Design review of the part shown in the three views and the two pictorial views. Dimensions are in mm from the part's minimum x, y and z. A direction names the side the tool comes from. Give positions to 0.01 mm unless a question says otherwise; leave off trailing zeros. Loops run counter-clockwise (first coordinate to the right, second up) from the corner with the lowest first, then second, coordinate; pieces in that order, holes last. Notation, with made-up numbers: (65, 56) -> (113, 56) arc R13 cw to (113, 70) -> close; hole circle Ø6 at (74.5, -13). An arc over 180 degrees is marked (long way). One line per question, with ' | ' between items. Start each with the question number.
(1) Wall thickness on probe 1 along Y at (x, z) = (20, 3.75); probe 2 along Y at (x, z) = (19, 2.5); probe 3 along X at (y, z) = (3.5, 1.5): over which ranges is each line inside the solid? List them lowest first.
(2) Consider section D-D (z = 8.75). Write out the cut boundary in (x, y), and give its area (3 significant figures).
(3) Draft analysis for pull direction Y (two halves, no side actions). For the marked faces 3, 4, 5 and 6, state which applies: +Y half, -Y half, draft (parallel to the pull), parting line (faces both ways), or undercut.
(4) Consider section A-A (z = 1.25). Write out the cut boundary in (x, y), and give its area (3 significant figures).
(5) Consider section C-C (y = 4). Write out the cut boundary in (x, z), and give its area (3 significant figures).
(6) Tool access review of the marked faces 1 and 2: name each direction out of +Z, -Z, +X, -X, +Y, -Y from which nothing blocks a thin tool from reaching the whole face with its end or side.
(7) Consider section B-B (x = 4). Write out the cut boundary in (y, z).
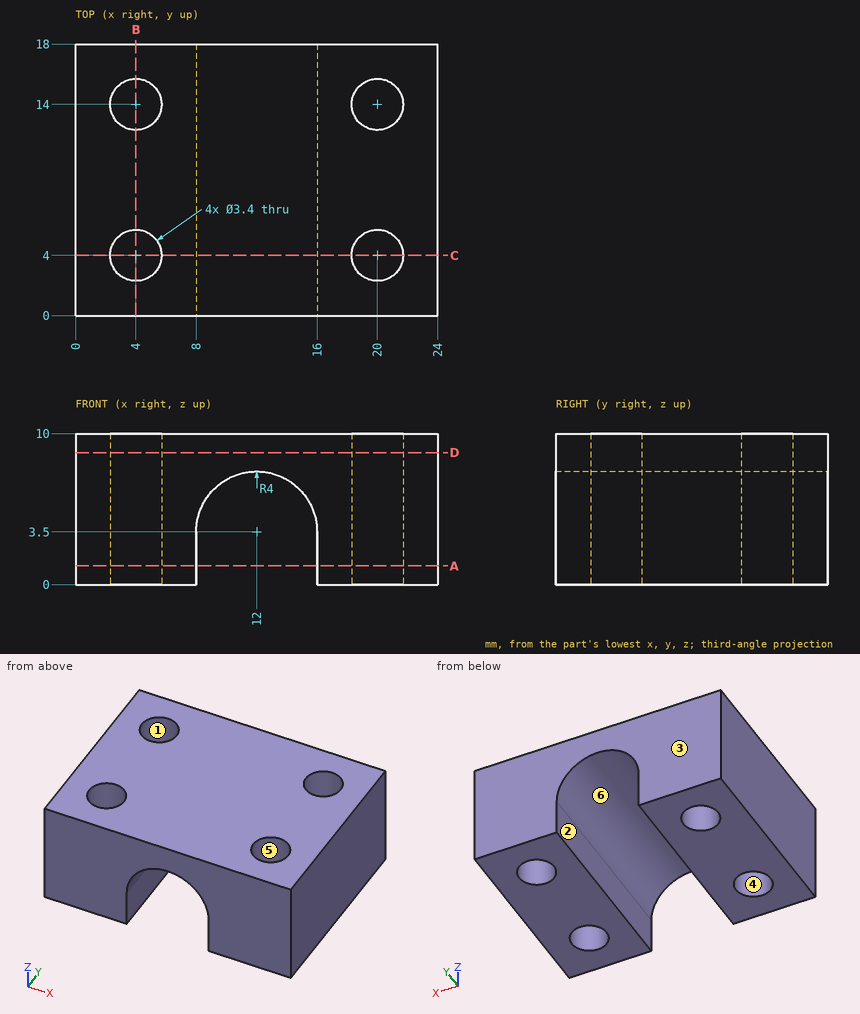
A:
1) probe 1: y = 0 to 2.3, 5.7 to 12.3, 15.7 to 18 | probe 2: y = 0 to 2.63, 5.37 to 12.63, 15.37 to 18 | probe 3: x = 0 to 2.38, 5.62 to 8, 16 to 18.38, 21.62 to 24
2) outline: (0, 0) -> (24, 0) -> (24, 18) -> (0, 18) -> close; hole circle Ø3.4 at (4, 4); hole circle Ø3.4 at (4, 14); hole circle Ø3.4 at (20, 4); hole circle Ø3.4 at (20, 14) | area: 396 mm^2
3) face 3: +Y half | face 4: undercut | face 5: undercut | face 6: draft
4) outline: (0, 0) -> (8, 0) -> (8, 18) -> (0, 18) -> close; (16, 0) -> (24, 0) -> (24, 18) -> (16, 18) -> close; hole circle Ø3.4 at (4, 4); hole circle Ø3.4 at (4, 14); hole circle Ø3.4 at (20, 4); hole circle Ø3.4 at (20, 14) | area: 252 mm^2
5) outline: (0, 0) -> (2.3, 0) -> (2.3, 10) -> (0, 10) -> close; (5.7, 0) -> (8, 0) -> (8, 3.5) arc R4 cw to (16, 3.5) -> (16, 0) -> (18.3, 0) -> (18.3, 10) -> (5.7, 10) -> close; (21.7, 0) -> (24, 0) -> (24, 10) -> (21.7, 10) -> close | area: 119 mm^2
6) face 1: +Z, -Z | face 2: -Z, +Y, -Y
7) outline: (0, 0) -> (2.3, 0) -> (2.3, 10) -> (0, 10) -> close; (5.7, 0) -> (12.3, 0) -> (12.3, 10) -> (5.7, 10) -> close; (15.7, 0) -> (18, 0) -> (18, 10) -> (15.7, 10) -> close
